Input: part model. Units: mm. Frame: model coordinates. Coordinates: 2 decimals unless noted, no trailing zeros. Order: outer loops, then holes, each group sorted by start corner. A loop starts at its lowest first (then second) coordinate and runs counter-clockwise, first axis right, second up.
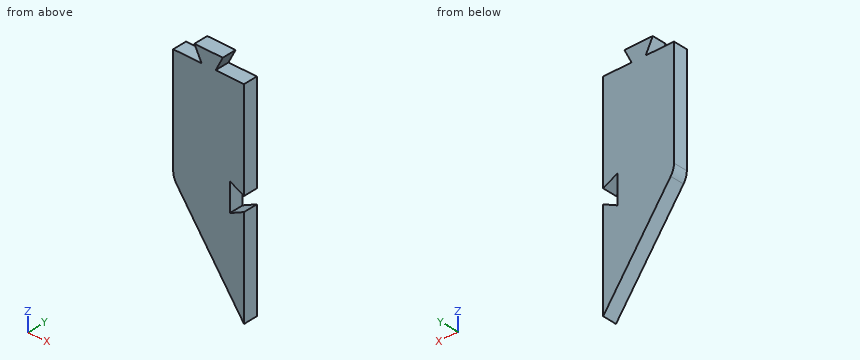
from build123d import *

# Parameters (mm, degrees)
EXTRUDE_1_DEPTH = 4


with BuildPart() as part:
    # Эскиз1 → Бобышка-Вытянуть1 (new body)
    with BuildSketch(Plane(origin=(0, 0, 0), x_dir=(1, 0, 0), z_dir=(0, 1, 0))):
        with BuildLine():
            Line((10, -17.5), (2, -17.5))
            Line((2, -17.5), (4, -21.5))
            Line((4, -21.5), (-4, -21.5))
            Line((-4, -21.5), (-2, -17.5))
            Line((-2, -17.5), (-10, -17.5))
            Line((-10, -17.5), (-10, 12.897674733))
            ThreePointArc((-10, 12.897674733), (-9.761477543, 14.423561888), (-9.068667356, 15.803865702))
            Line((-9.068667356, 15.803865702), (10, 42.5))
            Line((10, 42.5), (10, 14.5))
            Line((10, 14.5), (6, 16.5))
            Line((6, 16.5), (6, 8.5))
            Line((6, 8.5), (10, 10.5))
            Line((10, 10.5), (10, -17.5))
        make_face()
    extrude(amount=EXTRUDE_1_DEPTH)


solid = part.part
Item 1: Cut plane A-A on x = 3.25. Return loops of the section in (y, z).
Response values:
outline: (0, -33.05) - (4, -33.05) - (4, 17.5) - (0, 17.5) - close; (0, 20) - (4, 20) - (4, 21.5) - (0, 21.5) - close
Item 2: Ray query, probe 1 along X at (y, z) = (1.8, -10); probe 2 along Z at (x, y) = (2.5, 3.65); probe 3 along X at (y, z) = (1.5, -9). Return the intervals inside material, ascending.
Response values:
probe 1: x = -10 to 6, 9 to 10
probe 2: z = -32 to 17.5, 18.5 to 21.5
probe 3: x = -10 to 6, 7 to 10
Item 3: Pin query (flat end, axial travel): pin 1 Ø1.2 at (x, y) = (-6, 3) entering from +Z; pin 2 Ø1.5 at (x, z) = (2, -33) entering from +Y; pin 3 Ø5 at (x, z) = (-4, -17.5) entering from -Y. Return the tip coordinate at first contact, or that it passes through.
Response values:
pin 1: stops at z = 17.5
pin 2: passes through
pin 3: stops at y = 0
Item 4: Cut plane C-C on x = 0.5. Return loops of the section in (y, z), then the cut area to 3 significant figures.
Response values:
outline: (0, -29.2) - (4, -29.2) - (4, 21.5) - (0, 21.5) - close
area: 203 mm2
Item 5: Cut plane D-D on x = 8.25. Return loops of the section in (y, z) (3 decimals), then the cut area to 3 significant figures.
Response values:
outline: (0, -40.05) - (4, -40.05) - (4, -15.375) - (0, -15.375) - close; (0, -9.625) - (4, -9.625) - (4, 17.5) - (0, 17.5) - close
area: 207 mm2
Item 6: Cut plane B-B on y = 2.2. Return loops of the section in (x, z).
Response values:
outline: (-10, -12.9) arc R5 ccw to (-9.07, -15.8) - (10, -42.5) - (10, -14.5) - (6, -16.5) - (6, -8.5) - (10, -10.5) - (10, 17.5) - (2, 17.5) - (4, 21.5) - (-4, 21.5) - (-2, 17.5) - (-10, 17.5) - close
